Study the drawing (mm; zero at the part's minimum x, y, z) and answer. A direction names the side the tool comes from. Round coordinates to 2 decimals unless told otherwise and drop trailing zeros. Write each loop counter-clockwise with the first axis right and the second up, starting at its lowest first coordinate (ties: lowest second). Pieces come first, ordered by that corner, then holes. Notation, with made-up numbers: (48, 81.25) -> (100, 81.25) arc R34 ccw to (100, 114.25) -> close; hole circle Ø9 at (27.25, 56). An arc over 180 degrees is marked (long way). Write each question's results on one line, items separated by ' | '. Start each with the question number.
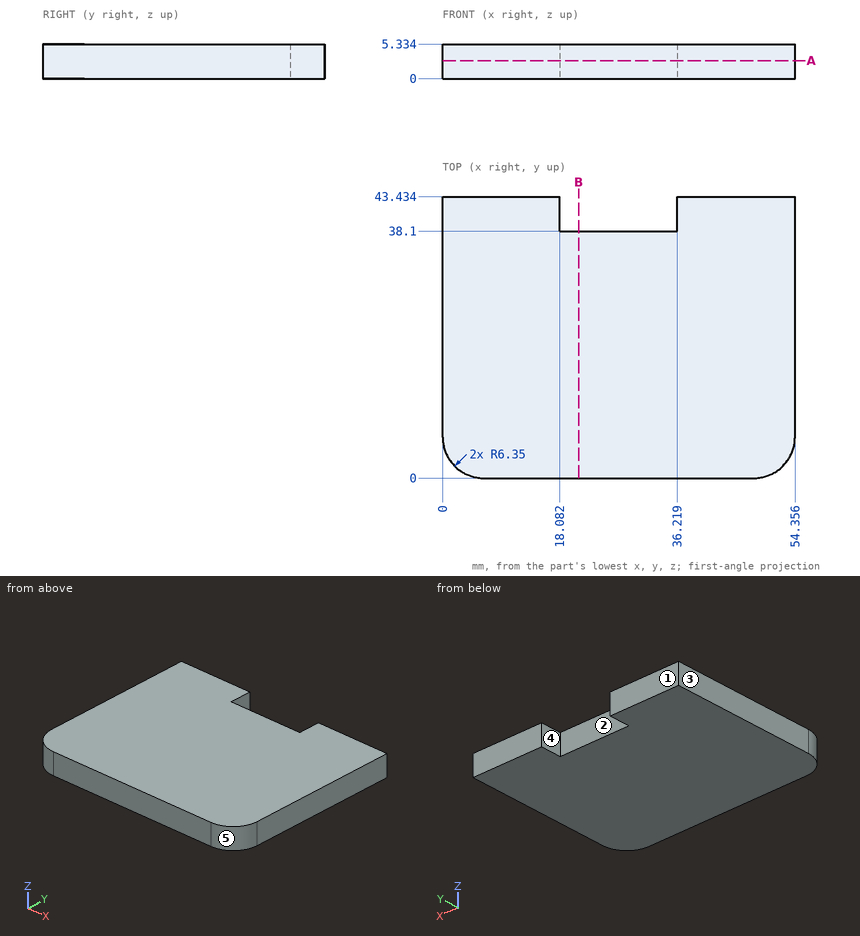
Q1. The part is cut by section B-B, the plane x = 21. Write down the section's boundary in (y, z).
Q2. This flat-tipped pin is pushed along its axis until it touches: pin 1 (3 mm diameter, centred on x = 24, z = 4, fed in from +Y). Where does it stop, or does it pass through?
Q3. Find the intervals of material crossed by line 1 (X direction, y = 41, z = 2.35); line 2 (Y direction, x = 26.5, z = 2.1); line 3 (X direction, y = 2, z = 0.25), in increasing order.
Q4. For the marked faces 1 and 2, determine the directions among +Z, -Z, +X, -X, +Y, -Y from which every point of the face is accessible in a straight line to the end or side of a thin tool.
Q5. Determine the mould class of the marked faces 3, 4 and 5 for opening direction X: pulls with the +X half, pulls with the -X half, needs draft (parallel to the pull), parting line crosses it, or undercut.
Q6. The part is cut by section A-A, the plane z = 2.75. Write down the section's boundary in (x, y), then the cut area to 3 significant figures.
Answers follow:
1) outline: (0, 0) -> (38.1, 0) -> (38.1, 5.33) -> (0, 5.33) -> close
2) pin 1: y = 38.1
3) line 1: 0 to 18.08, 36.22 to 54.36 | line 2: 0 to 38.1 | line 3: 1.72 to 52.63
4) face 1: +Z, -Z, +X, -X, +Y | face 2: +Z, -Z, +Y
5) face 3: pulls with the -X half | face 4: undercut | face 5: pulls with the +X half
6) outline: (0, 6.35) arc R6.35 ccw to (6.35, 0) -> (48.01, 0) arc R6.35 ccw to (54.36, 6.35) -> (54.36, 43.43) -> (36.22, 43.43) -> (36.22, 38.1) -> (18.08, 38.1) -> (18.08, 43.43) -> (0, 43.43) -> close | area: 2,250 mm^2
